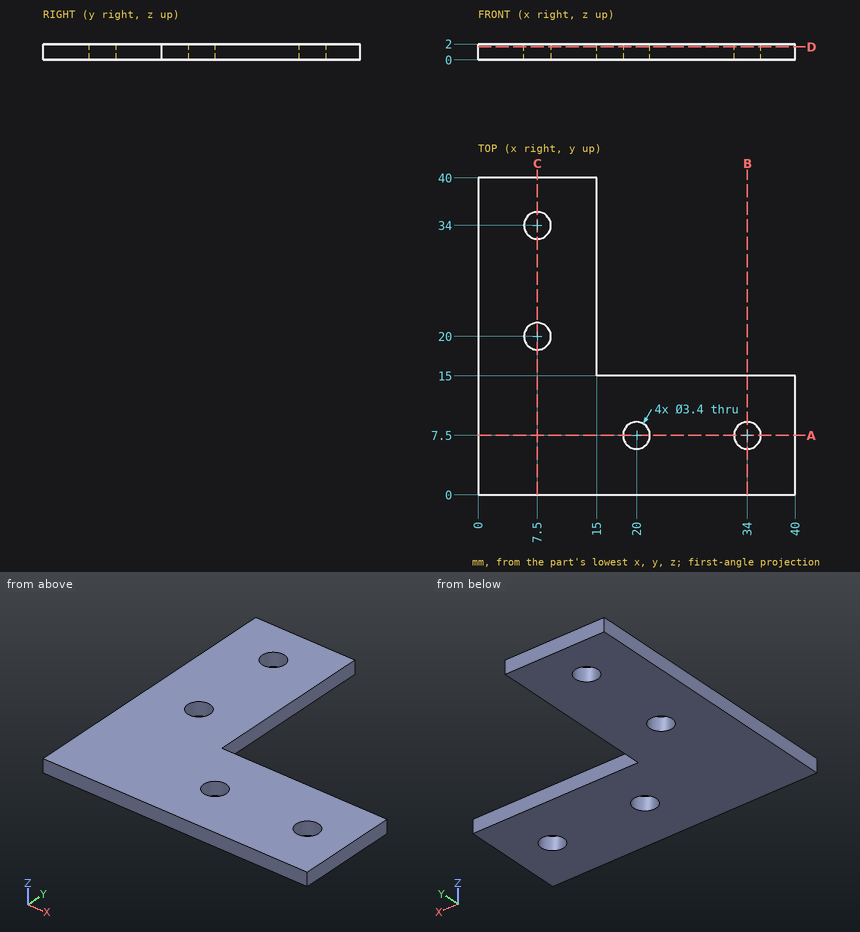
Input: dimensioned drawing with shaded views. Units: mm. Origin: part minimum x, y, z. Coordinates: 2 decimals unless noted, no trailing zeros. Order: outer loops, then holes, each group sorted by start corner. A loop starts at its lowest first (then second) coordinate and runs counter-clockwise, first axis right, second up.
1. Contact query for a flat-ended pin moving along its axis: P1, Ø0.6, axis at x = 30.5, z = 1, coming from the +Y side. Output: stop coordinate, or through.
Checked values:
P1: stops at y = 15
2. Cut plane A-A, the plane y = 7.5. Return loops of the section in (x, z).
Checked values:
outline: (0, 0) - (18.3, 0) - (18.3, 2) - (0, 2) - close; (21.7, 0) - (32.3, 0) - (32.3, 2) - (21.7, 2) - close; (35.7, 0) - (40, 0) - (40, 2) - (35.7, 2) - close
3. Ray query, line 1 along Y through (x, z) = (7.5, 1.3); line 2 along Y through (x, z) = (34, 1.1). Return the intervals inside material, ascending.
Checked values:
line 1: y = 0 to 18.3, 21.7 to 32.3, 35.7 to 40
line 2: y = 0 to 5.8, 9.2 to 15
4. Cut plane D-D, the plane z = 1.65. Return loops of the section in (x, y).
Checked values:
outline: (0, 0) - (40, 0) - (40, 15) - (15, 15) - (15, 40) - (0, 40) - close; hole circle Ø3.4 at (7.5, 20); hole circle Ø3.4 at (7.5, 34); hole circle Ø3.4 at (20, 7.5); hole circle Ø3.4 at (34, 7.5)
5. Cut plane B-B, the plane x = 34. Return loops of the section in (y, z), plus the area to 3 significant figures.
Checked values:
outline: (0, 0) - (5.8, 0) - (5.8, 2) - (0, 2) - close; (9.2, 0) - (15, 0) - (15, 2) - (9.2, 2) - close
area: 23.2 mm2
